Here's how the part is built. I have some questions about the finished solid (model axes, mm). A direction names the side the tool comes from. Round coordinates to 2 decimals unless told otherwise and drop trailing zeros. Write each loop counter-clockwise with the first axis right and the second up, starting at its lowest first coordinate (ties: lowest second). Pieces come first, ordered by that corner, then holes. Notation, with made-up numbers: (88, 22.5) -> (114, 22.5) arc R9 cw to (114, 31.5) -> close; hole circle Ø8 at (24.25, -36). An arc over 180 degrees is marked (long way). Answer as CSV lines item,"result".
from build123d import *

# Parameters (mm, degrees)
F1_DEPTH = 19.05
F2_W     = 4.7625
F2_H     = 31.75
F3_DEPTH = 25.4
F4_W     = 29.21
F4_H     = 9.017
F5_DEPTH = 24.638
F7_DEPTH = 6.858
F8_R     = 6.6675
F9_DEPTH = 25.4


with BuildPart() as f1:
    # F0 (on Front) → F1 (new body)
    with BuildSketch(Plane.XZ):
        with BuildLine():
            Line((0, 101.6), (0, 127))
            ThreePointArc((0, 127), (-32.870018728, 122.6725799387), (-63.5, 109.9852262806))
            Line((-63.5, 109.9852262806), (-54.102, 93.7074127911))
            ThreePointArc((-54.102, 93.7074127911), (-48.9873127514, 94.3385338445), (-44.9764745007, 91.1025616626))
            ThreePointArc((-44.9764745007, 91.1025616626), (-23.092636652, 98.9408415795), (0, 101.6))
        make_face()
        with BuildLine():
            Line((-108.204, 0), (-127, 0))
            ThreePointArc((-127, 0), (-122.6725799387, -32.870018728), (-109.9852262806, -63.5))
            Line((-109.9852262806, -63.5), (-87.9881810245, -50.8))
            ThreePointArc((-87.9881810245, -50.8), (-97.2316006056, -29.4716108088), (-101.38537, -6.600511341))
            ThreePointArc((-101.38537, -6.600511341), (-106.1932232408, -4.7450096164), (-108.204, 0))
        make_face()
        with BuildLine():
            Line((0, 0), (0, 101.6))
            ThreePointArc((0, 101.6), (-23.092636652, 98.9408415795), (-44.9764745007, 91.1025616626))
            ThreePointArc((-44.9764745007, 91.1025616626), (-44.3940895106, 89.5935242281), (-44.196, 87.9881810245))
            ThreePointArc((-44.196, 87.9881810245), (-45.0807682334, 84.6861810245), (-47.498, 82.2689492579))
            Line((-47.498, 82.2689492579), (0, 0))
        make_face()
        with BuildLine():
            Line((-87.9881810245, -50.8), (0, 0))
            Line((0, 0), (-94.996, 0))
            ThreePointArc((-94.996, 0), (-96.8549903836, -4.5932232408), (-101.38537, -6.600511341))
            ThreePointArc((-101.38537, -6.600511341), (-97.2316006056, -29.4716108088), (-87.9881810245, -50.8))
        make_face()
        with BuildLine():
            Line((-54.102, 93.7074127911), (-63.5, 109.9852262806))
            ThreePointArc((-63.5, 109.9852262806), (-89.8025612107, 89.8025612107), (-109.9852262806, 63.5))
            Line((-109.9852262806, 63.5), (-93.7074127911, 54.102))
            ThreePointArc((-93.7074127911, 54.102), (-89.5935242281, 57.2059104894), (-84.5020503216, 56.4088954993))
            ThreePointArc((-84.5020503216, 56.4088954993), (-71.8420489686, 71.8420489686), (-56.4088954993, 84.5020503216))
            ThreePointArc((-56.4088954993, 84.5020503216), (-57.2059104894, 89.5935242281), (-54.102, 93.7074127911))
        make_face()
        with BuildLine():
            Line((-93.7074127911, 54.102), (-109.9852262806, 63.5))
            ThreePointArc((-109.9852262806, 63.5), (-122.6725799387, 32.870018728), (-127, 0))
            Line((-127, 0), (-108.204, 0))
            ThreePointArc((-108.204, 0), (-106.1932232408, 4.7450096164), (-101.38537, 6.600511341))
            ThreePointArc((-101.38537, 6.600511341), (-98.138063951, 26.2960149824), (-91.1025616626, 44.9764745007))
            ThreePointArc((-91.1025616626, 44.9764745007), (-94.3385338445, 48.9873127514), (-93.7074127911, 54.102))
        make_face()
        with BuildLine():
            Line((-82.2689492579, 47.498), (0, 0))
            Line((0, 0), (-47.498, 82.2689492579))
            ThreePointArc((-47.498, 82.2689492579), (-52.4053432036, 81.5822705351), (-56.4088954993, 84.5020503216))
            ThreePointArc((-56.4088954993, 84.5020503216), (-71.8420489686, 71.8420489686), (-84.5020503216, 56.4088954993))
            ThreePointArc((-84.5020503216, 56.4088954993), (-82.2160400369, 54.0086140963), (-81.3841810245, 50.8))
            ThreePointArc((-81.3841810245, 50.8), (-81.6092068677, 49.0907590261), (-82.2689492579, 47.498))
        make_face()
        with BuildLine():
            Line((-94.996, 0), (0, 0))
            Line((0, 0), (-82.2689492579, 47.498))
            ThreePointArc((-82.2689492579, 47.498), (-86.1754937759, 44.44964718), (-91.1025616626, 44.9764745007))
            ThreePointArc((-91.1025616626, 44.9764745007), (-98.138063951, 26.2960149824), (-101.38537, 6.600511341))
            ThreePointArc((-101.38537, 6.600511341), (-96.8549903836, 4.5932232408), (-94.996, 0))
        make_face()
        with BuildLine():
            Line((-101.6, 0), (-108.204, 0))
            ThreePointArc((-108.204, 0), (-106.1932232408, -4.7450096164), (-101.38537, -6.600511341))
            ThreePointArc((-101.38537, -6.600511341), (-101.5463283236, -3.302), (-101.6, 0))
        make_face()
        with BuildLine():
            ThreePointArc((-101.38537, -6.600511341), (-96.8549903836, -4.5932232408), (-94.996, 0))
            Line((-94.996, 0), (-101.6, 0))
            ThreePointArc((-101.6, 0), (-101.5463283236, -3.302), (-101.38537, -6.600511341))
        make_face()
        with BuildLine():
            ThreePointArc((-101.38537, 6.600511341), (-106.1932232408, 4.7450096164), (-108.204, 0))
            Line((-108.204, 0), (-101.6, 0))
            ThreePointArc((-101.6, 0), (-101.5463283236, 3.302), (-101.38537, 6.600511341))
        make_face()
        with BuildLine():
            Line((-101.6, 0), (-94.996, 0))
            ThreePointArc((-94.996, 0), (-96.8549903836, 4.5932232408), (-101.38537, 6.600511341))
            ThreePointArc((-101.38537, 6.600511341), (-101.5463283236, 3.302), (-101.6, 0))
        make_face()
        with BuildLine():
            ThreePointArc((-91.1025616626, 44.9764745007), (-86.1754937759, 44.44964718), (-82.2689492579, 47.498))
            Line((-82.2689492579, 47.498), (-87.9881810245, 50.8))
            ThreePointArc((-87.9881810245, 50.8), (-89.5926999893, 47.9135482785), (-91.1025616626, 44.9764745007))
        make_face()
        with BuildLine():
            Line((-87.9881810245, 50.8), (-93.7074127911, 54.102))
            ThreePointArc((-93.7074127911, 54.102), (-94.3385338445, 48.9873127514), (-91.1025616626, 44.9764745007))
            ThreePointArc((-91.1025616626, 44.9764745007), (-89.5926999893, 47.9135482785), (-87.9881810245, 50.8))
        make_face()
        with BuildLine():
            ThreePointArc((-84.5020503216, 56.4088954993), (-89.5935242281, 57.2059104894), (-93.7074127911, 54.102))
            Line((-93.7074127911, 54.102), (-87.9881810245, 50.8))
            ThreePointArc((-87.9881810245, 50.8), (-86.2906999893, 53.6327800451), (-84.5020503216, 56.4088954993))
        make_face()
        with BuildLine():
            Line((-87.9881810245, 50.8), (-82.2689492579, 47.498))
            ThreePointArc((-82.2689492579, 47.498), (-81.6092068677, 49.0907590261), (-81.3841810245, 50.8))
            ThreePointArc((-81.3841810245, 50.8), (-82.2160400369, 54.0086140963), (-84.5020503216, 56.4088954993))
            ThreePointArc((-84.5020503216, 56.4088954993), (-86.2906999893, 53.6327800451), (-87.9881810245, 50.8))
        make_face()
        with BuildLine():
            Line((-47.498, 82.2689492579), (-50.8, 87.9881810245))
            ThreePointArc((-50.8, 87.9881810245), (-53.6327800451, 86.2906999893), (-56.4088954993, 84.5020503216))
            ThreePointArc((-56.4088954993, 84.5020503216), (-52.4053432036, 81.5822705351), (-47.498, 82.2689492579))
        make_face()
        with BuildLine():
            ThreePointArc((-44.196, 87.9881810245), (-44.3940895106, 89.5935242281), (-44.9764745007, 91.1025616626))
            ThreePointArc((-44.9764745007, 91.1025616626), (-47.9135482785, 89.5926999893), (-50.8, 87.9881810245))
            Line((-50.8, 87.9881810245), (-47.498, 82.2689492579))
            ThreePointArc((-47.498, 82.2689492579), (-45.0807682334, 84.6861810245), (-44.196, 87.9881810245))
        make_face()
        with BuildLine():
            ThreePointArc((-44.9764745007, 91.1025616626), (-48.9873127514, 94.3385338445), (-54.102, 93.7074127911))
            Line((-54.102, 93.7074127911), (-50.8, 87.9881810245))
            ThreePointArc((-50.8, 87.9881810245), (-47.9135482785, 89.5926999893), (-44.9764745007, 91.1025616626))
        make_face()
        with BuildLine():
            Line((-50.8, 87.9881810245), (-54.102, 93.7074127911))
            ThreePointArc((-54.102, 93.7074127911), (-57.2059104894, 89.5935242281), (-56.4088954993, 84.5020503216))
            ThreePointArc((-56.4088954993, 84.5020503216), (-53.6327800451, 86.2906999893), (-50.8, 87.9881810245))
        make_face()
    extrude(amount=F1_DEPTH)

    # F2 (on face) → F3 (cut)
    with BuildSketch(Plane.YZ):
        with Locations((-7.14375, 47.625)):
            Rectangle(F2_W, F2_H)
        with Locations((-11.90625, 47.625)):
            Rectangle(F2_W, F2_H)
        with Locations((-11.90625, 79.375)):
            Rectangle(F2_W, F2_H)
        with Locations((-7.14375, 79.375)):
            Rectangle(F2_W, F2_H)
    extrude(amount=-F3_DEPTH, mode=Mode.SUBTRACT)

    # F4 (on face) → F5 (join)
    with BuildSketch(Plane(origin=(0, 0, 0), x_dir=(0.8660254038, 0, 0.5), z_dir=(0.5, 0, -0.8660254038))):
        with Locations((-78.105, 9.525)):
            Rectangle(F4_W, F4_H)
        with Locations((-48.895, 9.525)):
            Rectangle(F4_W, F4_H)
    extrude(amount=F5_DEPTH)

    # F6 (on face) → F7 (cut)
    with BuildSketch(Plane.XZ.offset(19.05)):
        with BuildLine():
            ThreePointArc((-101.3812226563, -6.6639097176), (-96.808640371, -4.6366398561), (-94.9325, 0))
            Line((-94.9325, 0), (-101.6, 0))
            ThreePointArc((-101.6, 0), (-101.5452909343, -3.33375), (-101.3812226563, -6.6639097176))
        make_face()
        with BuildLine():
            ThreePointArc((-101.3812226563, -6.6639097176), (-101.5452909343, -3.33375), (-101.6, 0))
            Line((-101.6, 0), (-108.2675, 0))
            ThreePointArc((-108.2675, 0), (-106.2366398561, -4.791359629), (-101.3812226563, -6.6639097176))
        make_face()
        with BuildLine():
            Line((-108.2675, 0), (-101.6, 0))
            ThreePointArc((-101.6, 0), (-101.5452909343, 3.33375), (-101.3812226563, 6.6639097176))
            ThreePointArc((-101.3812226563, 6.6639097176), (-106.2366398561, 4.791359629), (-108.2675, 0))
        make_face()
        with BuildLine():
            Line((-101.6, 0), (-94.9325, 0))
            ThreePointArc((-94.9325, 0), (-96.808640371, 4.6366398561), (-101.3812226563, 6.6639097176))
            ThreePointArc((-101.3812226563, 6.6639097176), (-101.5452909343, 3.33375), (-101.6, 0))
        make_face()
        with BuildLine():
            ThreePointArc((-91.1306691458, 44.9194962242), (-86.1570617951, 44.3888722819), (-82.2139566448, 47.46625))
            Line((-82.2139566448, 47.46625), (-87.9881810245, 50.8))
            ThreePointArc((-87.9881810245, 50.8), (-89.6076765838, 47.8855332773), (-91.1306691458, 44.9194962242))
        make_face()
        with BuildLine():
            ThreePointArc((-91.1306691458, 44.9194962242), (-89.6076765838, 47.8855332773), (-87.9881810245, 50.8))
            Line((-87.9881810245, 50.8), (-93.7624054042, 54.13375))
            ThreePointArc((-93.7624054042, 54.13375), (-94.3993087426, 48.9688807706), (-91.1306691458, 44.9194962242))
        make_face()
        with BuildLine():
            Line((-93.7624054042, 54.13375), (-87.9881810245, 50.8))
            ThreePointArc((-87.9881810245, 50.8), (-86.2739265838, 53.659757657), (-84.4667594283, 56.4617264321))
            ThreePointArc((-84.4667594283, 56.4617264321), (-89.6079491136, 57.2677590855), (-93.7624054042, 54.13375))
        make_face()
        with BuildLine():
            Line((-87.9881810245, 50.8), (-82.2139566448, 47.46625))
            ThreePointArc((-82.2139566448, 47.46625), (-81.5478705777, 49.0743240168), (-81.3206810245, 50.8))
            ThreePointArc((-81.3206810245, 50.8), (-82.1600323157, 54.0385550603), (-84.4667594283, 56.4617264321))
            ThreePointArc((-84.4667594283, 56.4617264321), (-86.2739265838, 53.659757657), (-87.9881810245, 50.8))
        make_face()
        with BuildLine():
            ThreePointArc((-56.4577228186, 84.4694355027), (-52.4186754183, 81.525109972), (-47.4686565195, 82.2181248589))
            Line((-47.4686565195, 82.2181248589), (-50.8, 87.9881810245))
            ThreePointArc((-50.8, 87.9881810245), (-53.6577130389, 86.2751982405), (-56.4577228186, 84.4694355027))
        make_face()
        with BuildLine():
            Line((-54.1313434805, 93.7582371901), (-50.8, 87.9881810245))
            ThreePointArc((-50.8, 87.9881810245), (-47.8876568733, 89.6065417209), (-44.9238155794, 91.128539952))
            ThreePointArc((-44.9238155794, 91.128539952), (-48.9702785065, 94.3947024516), (-54.1313434805, 93.7582371901))
        make_face()
        with BuildLine():
            ThreePointArc((-56.4577228186, 84.4694355027), (-53.6577130389, 86.2751982405), (-50.8, 87.9881810245))
            Line((-50.8, 87.9881810245), (-54.1313434805, 93.7582371901))
            ThreePointArc((-54.1313434805, 93.7582371901), (-57.2630710525, 89.6068564428), (-56.4577228186, 84.4694355027))
        make_face()
        with BuildLine():
            Line((-50.8, 87.9881810245), (-47.4686565195, 82.2181248589))
            ThreePointArc((-47.4686565195, 82.2181248589), (-45.0299438344, 84.656837544), (-44.1373130391, 87.9881810245))
            ThreePointArc((-44.1373130391, 87.9881810245), (-44.3369289475, 89.6068564428), (-44.9238155794, 91.128539952))
            ThreePointArc((-44.9238155794, 91.128539952), (-47.8876568733, 89.6065417209), (-50.8, 87.9881810245))
        make_face()
    extrude(amount=-F7_DEPTH, mode=Mode.SUBTRACT)

    # F8 (on face) → F9 (cut)
    with BuildSketch(Plane.XZ.offset(19.05)):
        Circle(F8_R)
    extrude(amount=-F9_DEPTH, mode=Mode.SUBTRACT)


solid = f1.part
Item 1: Suppose I cut it at D-D, the plane z = -30.5. List the corners of the cut face in (x, y) for me.
Results found:
outline,"(-123.28, -19.05) -> (-52.83, -19.05) -> (-52.83, -14.03) -> (-21.99, -14.03) -> (-21.99, -5.02) -> (-52.83, -5.02) -> (-52.83, 0) -> (-123.28, 0) -> close"
Item 2: Will these pins go through, and if not, where does the flat tip stop? pin 1 (10 mm diameter, centred on x = -19, z = 10.5, fed in from +Y); pin 2 (3 mm diameter, centred on y = -9.5, z = 50.5, fed in from +X); pin 3 (5 mm diameter, centred on x = -88, y = -6.5, fed in from +Z); pin 4 (5 mm diameter, centred on x = -14, y = -7.5, fed in from +Z).
Results found:
pin 1,"stops at y = 0"
pin 2,"stops at x = -25.4"
pin 3,"stops at z = 93.91"
pin 4,"stops at z = 126.48"
Item 3: I need wall thicknesses on L1, parallel to Y at x = -98, z = 5.5; L2, parallel to Y at x = -51.5, z = -41; L3, parallel to X at y = -15.75, z = 53. Which ranges of each line are inside material? Lowest first, please.
Results found:
L1,"y = -12.19 to 0"
L2,"y = -14.03 to -5.02"
L3,"x = -115.41 to -94.28, -81.69 to 0"
Item 4: If we mould it in two halves opening along Z, with no side actions, what happens to faces 1 (the flat face through (-64, 0, 33)), 2 (the flat face through (-13, -14.288, 64)), 3 (the flat face through (-43.028, -9.588, -53.292))? For each: pulls with the +Z half, pulls with the -Z half, needs draft (parallel to the pull), parting line crosses it, or undercut.
Results found:
face 1,"needs draft"
face 2,"undercut"
face 3,"pulls with the -Z half"
Item 5: Suppose I cut it at C-C, the plane x = -15.5. List the corners of the cut face in (y, z) for me.
Results found:
outline,"(-19.05, -8.95) -> (0, -8.95) -> (0, 126.05) -> (-19.05, 126.05) -> close; hole (-14.29, 31.75) -> (-4.76, 31.75) -> (-4.76, 95.25) -> (-14.29, 95.25) -> close"
Item 6: Suppose I cut it at A-A, the plane z = -54. List the corners of the cut face in (x, y) for me, then the cut area to 3 significant figures.
Results found:
outline,"(-114.95, -19.05) -> (-93.53, -19.05) -> (-93.53, 0) -> (-114.95, 0) -> close; (-75.88, -14.03) -> (-44.25, -14.03) -> (-44.25, -5.02) -> (-75.88, -5.02) -> close"
area,"693 mm²"
Item 7: For faces 4 (the flat face through (-74.2, -9.5, -56.9)), 5 (the flat face through (-23.6, -9.5, -27.7)), 6 (the flat face through (-13, -9, 95.25)), 7 (the flat face through (-51, -12.192, 88)), which set-ups out of +Z, -Z, +X, -X, +Y, -Y let a thin tool reach every point of the face, with its end or its side?
Results found:
face 4,"-Z, +Y, -Y"
face 5,"+X, +Y, -Y"
face 6,"+X"
face 7,"-Y"
